from build123d import *

# Parameters (mm, degrees)
BOSS_EXTRUDE1_DEPTH = 3.175
SKETCH2_W           = 29.21
SKETCH2_H           = 5.9436
CUT_EXTRUDE2_DEPTH  = 4.064


with BuildPart() as part:
    # Sketch1 → Boss-Extrude1 (new body)
    with BuildSketch(Plane(origin=(0, 0, 0), x_dir=(1, 0, 0), z_dir=(0, 1, 0))):
        Polygon((-54.3052, -23.114), (-37.2872, -23.114), (-37.2872, -19.939), (-20.2692, -19.939), (-20.2692, -23.114), (-3.2512, -23.114), (-3.2512, -19.939), (13.7668, -19.939), (13.7668, -23.114), (30.7848, -23.114), (30.7848, -19.939), (47.8028, -19.939), (47.8028, -23.114), (60.5028, -23.114), (60.5028, -19.939), (64.4398, -19.939), (64.4398, -23.114), (71.3232, -23.114), (71.3232, 23.114), (64.4398, 23.114), (64.4398, 19.939), (60.5028, 19.939), (60.5028, 23.114), (47.8028, 23.114), (47.8028, 19.939), (30.7848, 19.939), (30.7848, 23.114), (13.7668, 23.114), (13.7668, 19.939), (-3.2512, 19.939), (-3.2512, 23.114), (-20.2692, 23.114), (-20.2692, 19.939), (-37.2872, 19.939), (-37.2872, 23.114), (-54.3052, 23.114), (-54.3052, 19.939), (-71.3232, 19.939), (-71.3232, -19.939), (-54.3052, -19.939), align=None)
    extrude(amount=BOSS_EXTRUDE1_DEPTH)

    # Sketch2 → Cut-Extrude2 (cut)
    with BuildSketch(Plane(origin=(0, 3.175, 0), x_dir=(1, 0, 0), z_dir=(0, 1, 0))):
        with Locations((-56.7182, 13.3604)):
            Rectangle(SKETCH2_W, SKETCH2_H)
    extrude(amount=-CUT_EXTRUDE2_DEPTH, mode=Mode.SUBTRACT)


solid = part.part
Input: part model. Units: mm. Frame: model coordinates. A direction names the side the tool comes from. Give positions to 0.01 mm unless a question says otherwise; leave off trailing zeros. Write each loop counter-clockwise with the first axis right and the second up, starting at its lowest first coordinate (ties: lowest second). Pieces come first, ordered by that corner, then holes. Notation, with made-up numbers: M 38,25 L 64,25 A22 cw 64,58 Z; hole C 7.25,-21 d8. An arc over 180 degrees is marked long. Use one line per item in the form item = value.
1. Mould query, pull axis Z, two halves, no side actions, for faces 1 (the face through (64.44, 2, 22)), 2 (the face through (-42.113, 2, -13)), 3 (the face through (-46, 2, -23.114)). Classes: released by +Z, released by -Z, zero draft, split by the parting line, or undercut.
Outcome:
face_1 = zero draft
face_2 = undercut
face_3 = released by -Z
2. Reachability of faces 4 (the face through (-29, 2, 19.939)), 5 (the face through (-54.305, 2, -22)), 6 (the face through (64.44, 2, -22)) from +Z, -Z, +X, -X, +Y, -Y: full face, straight path, thin tool, end or side. Return the list, or none.
Outcome:
face_4 = +Z, +Y, -Y
face_5 = -Z, -X, +Y, -Y
face_6 = -Z, +Y, -Y
3. First-contact query: P1, Ø1.6, axis at x = 62, y = 2.5, coming from the -Z side; P2, Ø1.6, axis at x = 40.5, y = 2, coming from the +Z side; P3, Ø1, axis at y = 2, z = -21.5, coming from the -X side. Flat tips, straight axial feed; report the tip coordinate or a pass-through.
Outcome:
P1 = -19.94
P2 = 19.94
P3 = -54.31
4. Cut plane A-A on x = -44. Return loops of the section in (y, z) (3 decimals), and give its area (3 significant figures).
Outcome:
outline = M 0,-23.114 L 3.175,-23.114 L 3.175,-16.332 L 0,-16.332 Z; M 0,-10.389 L 3.175,-10.389 L 3.175,23.114 L 0,23.114 Z
area = 128 mm²
5. Cut plane C-C on x = -22. Return loops of the section in (y, z) (3 decimals).
Outcome:
outline = M 0,-19.939 L 3.175,-19.939 L 3.175,19.939 L 0,19.939 Z
6. Ray query, L1, parallel to Z at x = -49, y = 2.4; L2, parallel to Z at x = -57, y = 1.95; L3, parallel to Z at x = -32.5, y = 2.4. Return the intervals inside material, ascending.
Outcome:
L1 = -23.11 to -16.33, -10.39 to 23.11
L2 = -19.94 to -16.33, -10.39 to 19.94
L3 = -19.94 to 19.94
7. Cut plane B-B on z = -12.5. Return loops of the section in (x, y) (3 decimals), and give its area (3 significant figures).
Outcome:
outline = M -42.113,0 L 71.323,0 L 71.323,3.175 L -42.113,3.175 Z
area = 360 mm²
